```python
from build123d import *

# Parameters (mm, degrees)
SKETCH1_R           = 3.2639
BOSS_EXTRUDE1_DEPTH = 3.175
BOSS_EXTRUDE2_DEPTH = 0.79375


with BuildPart() as part:
    # Sketch1 → Boss-Extrude1 (new body)
    with BuildSketch(Plane(origin=(0, 0, 0), x_dir=(0, 0, -1), z_dir=(1, 0, 0))):
        with BuildLine():
            Line((172.062748254, 15.053539887), (172.72, 0))
            ThreePointArc((172.72, 0), (177.8, -5.08), (182.88, 0))
            Line((182.88, 0), (182.198650149, 15.716317735))
            ThreePointArc((182.198650149, 15.716317735), (176.791948401, 20.565465387), (172.062748254, 15.053539887))
        make_face()
        with Locations((177.8, 0)):
            Circle(SKETCH1_R, mode=Mode.SUBTRACT)
        with Locations((177.123417321, 15.496291061)):
            Circle(SKETCH1_R, mode=Mode.SUBTRACT)
    extrude(amount=BOSS_EXTRUDE1_DEPTH)

    # Sketch2 → Boss-Extrude2 (add)
    with BuildSketch(Plane.ZY):
        Polygon((-182.539325075, 7.858158868), (-182.60808341, 6.272148609), (-172.465486686, 5.829313272), (-172.326859023, 9.004408754), (-182.470566739, 9.444169127), align=None)
    extrude(amount=BOSS_EXTRUDE2_DEPTH)


solid = part.part
```
Read the model definition and answer for the solid it produces. Units are mm, in the model's axes. Round coordinates to 2 decimals unless told otherwise and drop trailing zeros. Loops run counter-clockwise (first coordinate to the right, second up) from the corner with the lowest first, then second, coordinate; pieces in that order, holes last. Notation, with made-up numbers: (1.25, 65) -> (15.25, 65) arc R22 ccw to (15.25, 76) -> close; hole circle Ø1 at (36, -13). An arc over 180 degrees is marked (long way). One line per item, written item: value.
1) A cutting plane is placed at A-A (y = -2). Determine the outline of the cut face in (x, z) (3 decimals).
Answer list:
outline: (0, -182.47) -> (3.175, -182.47) -> (3.175, -180.379) -> (0, -180.379) -> close; (0, -175.221) -> (3.175, -175.221) -> (3.175, -173.13) -> (0, -173.13) -> close
2) Consider L1, parallel to Y at x = 1.1, z = -178.75; L2, parallel to Y at x = 1.85, z = -177.8; L3, parallel to X at y = 9.25, z = -174.25 (3 decimals). Determine where each line is inside the solid, lowest interval first. Write a range as [from, to].
Answer list:
L1: y = [-4.99, -3.12], [3.12, 12.67], [18.33, 20.31]
L2: y = [-5.08, -3.26], [3.26, 12.3], [18.69, 20.53]
L3: x = [0, 3.175]
3) A cutting plane is placed at C-C (x = 0.3). Determine the outline of the cut face in (y, z), and give its area (3 significant figures).
Answer list:
outline: (0, -182.88) -> (15.72, -182.2) arc R5.08 ccw (long way) to (15.05, -172.06) -> (0, -172.72) arc R5.08 ccw to start; hole circle Ø6.53 at (0, -177.8); hole circle Ø6.53 at (15.5, -177.12)
area: 172 mm²
4) The mould has two halves that part along Z. Classify faces 1 (the face through (1.565, -1.25, -180.815)), 2 (the face through (1.57, 20.57, -176.91)), 3 (the face through (-0.794, 8, -178)): pulls with the +Z half, pulls with the -Z half, needs draft (parallel to the pull), parting line crosses it, or undercut.
Answer list:
face 1: undercut
face 2: parting line crosses it
face 3: needs draft
5) A cutting plane is placed at D-D (z = -179.5). Determine the outline of the cut face in (x, y) (3 decimals), and give its area (3 significant figures).
Answer list:
outline: (-0.794, 6.136) -> (0, 6.136) -> (0, 2.786) -> (3.175, 2.786) -> (3.175, 13.259) -> (0, 13.259) -> (0, 9.315) -> (-0.794, 9.315) -> close; (0, -4.787) -> (3.175, -4.787) -> (3.175, -2.786) -> (0, -2.786) -> close; (0, 17.733) -> (3.175, 17.733) -> (3.175, 19.986) -> (0, 19.986) -> close
area: 49.3 mm²
6) A cutting plane is placed at B-B (z = -177.75). Determine the outline of the cut face in (x, y) (1 decimal).
Answer list:
outline: (-0.8, 6.1) -> (0, 6.1) -> (0, 3.3) -> (3.2, 3.3) -> (3.2, 12.3) -> (0, 12.3) -> (0, 9.2) -> (-0.8, 9.2) -> close; (0, -5.1) -> (3.2, -5.1) -> (3.2, -3.3) -> (0, -3.3) -> close; (0, 18.7) -> (3.2, 18.7) -> (3.2, 20.5) -> (0, 20.5) -> close
7) A flat-ended cylindrical pin translates along its axis: P1, Ø5, axis at y = 17, z = -178, coming from the -X side. Find the tip coordinate at first contact, or state that the pin passes through.
Answer list:
P1: stops at x = 0
